Here's how the part is built. I have some questions about the finished solid (model axes, mm). A direction names the side the tool comes from. Round coordinates to 2 decimals unless told otherwise and drop trailing zeros. Write each loop counter-clockwise with the first axis right and the second up, starting at its lowest first coordinate (ties: lowest second). Pieces come first, ordered by that corner, then holes. Notation, with made-up numbers: (30, 88.5) -> (79, 88.5) arc R17 ccw to (79, 119.5) -> close; hole circle Ø8 at (28, -29). An arc over 180 degrees is marked (long way). Put each result on its own line as item: value. Start each with the question number.
1. Suppose I cut it at B-B (y = -5.5). Count the separate pieces of the cut face and the enclosed holes in it, then the cut area to 3 significant figures.
2. Suppose I cut it at A-A (x = 0). Please give me the cut outline in (y, z), then the cut area to 3 significant figures.
3. Suppose I cut it at D-D (x = -22). Please give me the cut outline in (y, z), then the cut area to 3 significant figures.
4. I need wall thicknesses on probe 1 along Y at (x, z) = (-9.5, 10.5); probe 2 along Y at (x, z) = (-28.5, -7.5); probe 3 along X at (y, z) = (5.25, 6). Which ranges of each line are inside material? Lowest first, please. Write a range as from..to.
5. We'd pull the mould along Z, two halves only. Please class faces 1 (the face through (0, -5, 40)), 2 (the face through (-1, 14, 3)), 3 (the face through (-30, -10, -18)): +Z half, -Z half, draft (parallel to the pull), parting line (faces both ways), or undercut.
6. For pin 1 (1.5 mm diameter, centred on x = 32.5, z = 2, fed in from -Y); pin 2 (1.5 mm diameter, centred on y = -4.5, z = -12.5, fed in from -X); pin 3 (6 mm diameter, centred on y = -3.5, z = -27.5, fed in from -X), each with a flat end and sliding along its axis, tell me the tip position at first contact or that it passes through.
7. Suppose I cut it at C-C (z = 37). Please give me the cut outline in (x, y), then the cut area to 3 significant figures.
8. Which directions (+Z, -Z, +X, -X, +Y, -Y) give clear straight access to the entire face, cutting with the end or side of a thin tool? Please do faces 4 (the face through (0, -10, 35)), 5 (the face through (-26, 0, -14)).
```python
from build123d import *

# Parameters (mm, degrees)
SKETCH1_R                = 37.5
BOSS_EXTRUDE1_DEPTH      = 14
CUT_EXTRUDE2_START       = -14
CUT_EXTRUDE2_DEPTH       = 14
SKETCH4_R                = 45
SKETCH4_R_2              = 37.5
BOSS_EXTRUDE2_DEPTH      = 14
SKETCH6_R                = 45
BOSS_EXTRUDE3_DEPTH      = 2
SKETCH7_R                = 1.75
CUT_EXTRUDE3_DEPTH       = 66.620118866
CIRPATTERN2_COUNT        = 3
BOSS_EXTRUDE4_DEPTH      = 10
FILLET1_R                = 1
CIRPATTERN3_COUNT        = 3
FILLET1_OF_CIRPATTERN3_R = 1
CUT_EXTRUDE4_DEPTH       = 69.01470446
FILLET2_R                = 1
SKETCH15_R               = 45
BOSS_EXTRUDE5_DEPTH      = 2


# Read off the part's stored shape, not the designer's step: Cut-Extrude2
with BuildPart() as part:
    # Sketch1 → Boss-Extrude1 (new body)
    with BuildSketch(Plane(origin=(0, 0, 0), x_dir=(1, 0, 0), z_dir=(0, 1, 0))):
        with Locations(Location((0, 0, 0), (0, 0, 270))):
            Circle(SKETCH1_R)
    extrude(amount=BOSS_EXTRUDE1_DEPTH)

    # Cut-Extrude2 outline → Cut-Extrude2 (cut)
    with BuildSketch(Plane(origin=(0, 14, 0), x_dir=(1, 0, 0), z_dir=(0, 1, 0)).offset(CUT_EXTRUDE2_START)):
        with BuildLine():
            ThreePointArc((-24.104535363, -28.726666617), (0, -24.760936498), (24.104535363, -28.726666617))
            ThreePointArc((24.104535363, -28.726666617), (32.475952642, -18.75), (36.930290738, -6.511806663))
            ThreePointArc((36.930290738, -6.511806663), (21.443600029, 12.380468249), (12.825755375, 35.238473279))
            ThreePointArc((12.825755375, 35.238473279), (0, 37.5), (-12.825755375, 35.238473279))
            ThreePointArc((-12.825755375, 35.238473279), (-21.443600029, 12.380468249), (-36.930290738, -6.511806663))
            ThreePointArc((-36.930290738, -6.511806663), (-32.475952642, -18.75), (-24.104535363, -28.726666617))
        make_face()
    extrude(amount=CUT_EXTRUDE2_DEPTH, mode=Mode.SUBTRACT)

    # Sketch4 → Boss-Extrude2 (add)
    with BuildSketch(Plane(origin=(0, 0, 0), x_dir=(1, 0, 0), z_dir=(0, 1, 0))):
        with Locations(Location((0, 0, 0), (0, 0, 270))):
            Circle(SKETCH4_R)
        Circle(SKETCH4_R_2, mode=Mode.SUBTRACT)
    extrude(amount=BOSS_EXTRUDE2_DEPTH)

    # Sketch6 → Boss-Extrude3 (add)
    with BuildSketch(Plane(origin=(0, 14, 0), x_dir=(1, 0, 0), z_dir=(0, 1, 0))):
        with Locations(Location((0, 0, 0), (0, 0, 270))):
            Circle(SKETCH6_R)
        with BuildLine():
            ThreePointArc((-28.952849653, 1.653026611), (-25.11473671, -14.5), (-13.044861788, -25.900416617))
            ThreePointArc((-13.044861788, -25.900416617), (0, -24.760936498), (13.044861788, -25.900416617))
            ThreePointArc((13.044861788, -25.900416617), (25.11473671, -14.5), (28.952849653, 1.653026611))
            ThreePointArc((28.952849653, 1.653026611), (21.443600029, 12.380468249), (15.907987865, 24.247390006))
            ThreePointArc((15.907987865, 24.247390006), (0, 29), (-15.907987865, 24.247390006))
            ThreePointArc((-15.907987865, 24.247390006), (-21.443600029, 12.380468249), (-28.952849653, 1.653026611))
        make_face(mode=Mode.SUBTRACT)
    extrude(amount=BOSS_EXTRUDE3_DEPTH)

    # Sketch7 → Cut-Extrude3 (cut, through all)
    with BuildSketch(Plane(origin=(0, 16, 0), x_dir=(1, 0, 0), z_dir=(0, 1, 0))):
        with Locations(Location((0, 32, 0), (0, 0, 270))):
            Circle(SKETCH7_R)
    cut_extrude3 = extrude(amount=-CUT_EXTRUDE3_DEPTH, mode=Mode.SUBTRACT)

    # CirPattern2: Cut-Extrude3 ×3 about axis
    cirpattern2_axis = Axis((0, 0, 0), (0, 1, 0))
    for i in range(1, CIRPATTERN2_COUNT):
        add(cut_extrude3.rotate(cirpattern2_axis, i * 360 / CIRPATTERN2_COUNT), mode=Mode.SUBTRACT)

    # Sketch13 → Boss-Extrude4 (add)
    with BuildSketch(Plane.XZ):
        with BuildLine():
            ThreePointArc((-22.11228446, 33.332369792), (0, 29.760936498), (22.11228446, 33.332369792))
            ThreePointArc((22.11228446, 33.332369792), (0, 40), (-22.11228446, 33.332369792))
        make_face()
    boss_extrude4 = extrude(amount=BOSS_EXTRUDE4_DEPTH)

    # Fillet1
    fillet1_edges = [part.edges().sort_by_distance(p)[0] for p in [
        (22.11228446, -5, 33.332369792),
        (-22.11228446, -5, 33.332369792),
    ]]
    fillet(fillet1_edges, radius=FILLET1_R)

    # CirPattern3: Boss-Extrude4 ×3 about axis
    cirpattern3_axis = Axis((0, 0, 0), (0, 1, 0))
    for i in range(1, CIRPATTERN3_COUNT):
        add(boss_extrude4.rotate(cirpattern3_axis, i * 360 / CIRPATTERN3_COUNT))

    # Fillet1 of CirPattern3
    fillet1_of_cirpattern3_edges = [part.edges().sort_by_distance(p)[0] for p in [
        (17.810536778, -5, -35.815984974),
        (39.922821238, -5, 2.483615182),
        (-39.922821238, -5, 2.483615182),
        (-17.810536778, -5, -35.815984974),
    ]]
    fillet(fillet1_of_cirpattern3_edges, radius=FILLET1_OF_CIRPATTERN3_R)

    # Sketch14 → Cut-Extrude4 (cut, through all)
    with BuildSketch(Plane.XZ.offset(-14)):
        with BuildLine():
            Line((-33.206244265, 32.485097805), (-44.736042076, 12.514902195))
            ThreePointArc((-44.736042076, 12.514902195), (-21.443600029, -12.380468249), (-11.529797811, -45))
            Line((-11.529797811, -45), (11.529797811, -45))
            ThreePointArc((11.529797811, -45), (21.443600029, -12.380468249), (44.736042076, 12.514902195))
            Line((44.736042076, 12.514902195), (33.206244265, 32.485097805))
            ThreePointArc((33.206244265, 32.485097805), (0, 24.760936498), (-33.206244265, 32.485097805))
        make_face()
    extrude(amount=CUT_EXTRUDE4_DEPTH, mode=Mode.SUBTRACT)

    # Fillet2
    fillet2_edges = [part.edges().sort_by_distance(p)[0] for p in [
        (43.466885988, 7, 11.646021745),
        (11.64769231, 7, -43.466438362),
        (-31.819193678, 7, 31.820416617),
        (31.819193678, 7, 31.820416617),
        (-11.64769231, 7, -43.466438362),
        (-43.466885988, 7, 11.646021745),
    ]]
    fillet(fillet2_edges, radius=FILLET2_R)

    # Sketch15 → Boss-Extrude5 (add)
    with BuildSketch(Plane.XZ.offset(-14)):
        with Locations(Location((0, 0, 0), (0, 0, 253.108257002))):
            Circle(SKETCH15_R)
    extrude(amount=-BOSS_EXTRUDE5_DEPTH)


solid = part.part
```
Verdict:
1. separate pieces: 3
1. enclosed holes: 0
1. area: 911 mm^2
2. outline: (-10, 29.76) -> (0, 29.76) -> (0, 24.76) -> (14, 24.76) -> (14, -45) -> (16, -45) -> (16, 45) -> (0, 45) -> (0, 40) -> (-10, 40) -> close
2. area: 566 mm^2
3. outline: (-10, -33.41) -> (0, -33.41) -> (0, -39.26) -> (16, -39.26) -> (16, 39.26) -> (0, 39.26) -> (0, 28.05) -> (14, 28.05) -> (14, -11.43) -> (0, -11.43) -> (0, -22.43) -> (-10, -22.43) -> close
3. area: 813 mm^2
4. probe 1: y = 14..16
4. probe 2: y = 0..16
4. probe 3: x = -44.6..-36.35, 36.35..44.6
5. face 1: +Z half
5. face 2: undercut
5. face 3: draft
6. pin 1: stops at y = 0
6. pin 2: stops at x = -38.24
6. pin 3: stops at x = -31.62
7. outline: (-25.61, 0) -> (-15.2, 0) -> (-15.2, -10) -> (15.2, -10) -> (15.2, 0) -> (25.61, 0) -> (25.61, 16) -> (-25.61, 16) -> close
7. area: 1,120 mm^2
8. face 4: +Z, -Z, +X, -X, -Y
8. face 5: -Y
